Autodesk Inventor part; units mm, degrees
ref_plane "YZ Plane" through (0, 0, 0) normal (1, 0, 0) x (0, 1, 0)
ref_plane "XZ Plane" through (0, 0, 0) normal (0, 1, 0) x (-1, 0, 0)
ref_plane "XY Plane" through (0, 0, 0) normal (0, 0, 1) x (1, 0, 0)
sketch "Sketch1" plane through (0, 0, 0) normal (0, 0, 1) x (1, 0, 0)
  line L0 (-212.471, -44.069) -> (212.471, -44.069)
  line L1 (212.471, -44.069) -> (212.471, 44.069)
  line L2 (212.471, 44.069) -> (-212.471, 44.069)
  line L3 (-212.471, 44.069) -> (-212.471, -44.069)
  line L4 (-212.471, -44.069) -> (212.471, 44.069) construction
  line L5 (212.471, -44.069) -> (-212.471, 44.069) construction
  point P0 (0, 0)
  dimension "d0" = 424.942
  dimension "d1" = 88.138
extrude "Extrusion1" add sketch "Sketch1" along normal blind 1.651
sketch "SMA" plane through (0, 0, 1.651) normal (0, 0, 1) x (1, 0, 0)
  line L0 (-209.423, -35.814) -> (209.423, -35.814) construction
  line L1 (209.423, -35.814) -> (209.423, 35.814) construction
  line L2 (209.423, 35.814) -> (-209.423, 35.814) construction
  line L3 (-209.423, 35.814) -> (-209.423, -35.814) construction
  line L4 (212.471, 44.069) -> (-212.471, 44.069) construction
  line L5 (212.471, -44.069) -> (212.471, 44.069) construction
  line L6 (-212.471, 44.069) -> (-212.471, -44.069)
  line L7 (-212.471, -44.069) -> (212.471, -44.069)
  line L8 (-222.5982, 0) -> (228.0899, 0) construction
  line L9 (0, 79.8165) -> (0, -88.5526) construction
  line L10 (-181.2798, 19.5533) -> (-181.2798, 0.2592) construction
  line L11 (-189.2532, 10.414) -> (-170.7489, 10.414) construction
  arc A0 (-184.023, 8.669) -> (-184.023, 12.159) centre (-181.2798, 10.414) ccw
  line L12 (-184.023, 12.159) -> (-184.023, 8.669)
  line L13 (-145.923, 12.159) -> (-145.923, 8.669)
  arc A1 (-145.923, 8.669) -> (-145.923, 12.159) centre (-143.1798, 10.414) ccw
  line L14 (-184.023, -13.241) -> (-184.023, -16.731)
  arc A2 (-184.023, -16.731) -> (-184.023, -13.241) centre (-181.2798, -14.986) ccw
  line L15 (-145.923, -13.241) -> (-145.923, -16.731)
  arc A3 (-145.923, -16.731) -> (-145.923, -13.241) centre (-143.1798, -14.986) ccw
  line L16 (-120.523, 12.159) -> (-120.523, 8.669)
  arc A4 (-120.523, 8.669) -> (-120.523, 12.159) centre (-117.7798, 10.414) ccw
  arc A5 (-120.523, -16.731) -> (-120.523, -13.241) centre (-117.7798, -14.986) ccw
  line L17 (-120.523, -13.241) -> (-120.523, -16.731)
  line L18 (-95.123, 12.159) -> (-95.123, 8.669)
  arc A6 (-95.123, 8.669) -> (-95.123, 12.159) centre (-92.3798, 10.414) ccw
  arc A7 (-95.123, -16.731) -> (-95.123, -13.241) centre (-92.3798, -14.986) ccw
  line L19 (-95.123, -13.241) -> (-95.123, -16.731)
  line L20 (-69.723, 12.159) -> (-69.723, 8.669)
  arc A8 (-69.723, 8.669) -> (-69.723, 12.159) centre (-66.9798, 10.414) ccw
  arc A9 (-69.723, -16.731) -> (-69.723, -13.241) centre (-66.9798, -14.986) ccw
  line L21 (-69.723, -13.241) -> (-69.723, -16.731)
  point P0 (0, 0)
  point P1 (-178.0286, 10.414)
  point P2 (-139.9286, 10.414)
  point P3 (-178.0286, -14.986)
  point P4 (-139.9286, -14.986)
  point P5 (-114.5286, 10.414)
  point P6 (-114.5286, -14.986)
  point P7 (-89.1286, 10.414)
  point P8 (-89.1286, -14.986)
  point P9 (-63.7286, 10.414)
  point P10 (-63.7286, -14.986)
  point P11 (-63.7286, -14.986)
  dimension "d4" = 8.255
  dimension "d5" = 3.048
  dimension "d7" = 8.255
  dimension "d8" = 3.048
  dimension "d11" = 6.5024
  dimension "d12" = 5.9944
  dimension "d13" = 25.4
  dimension "d14" = 25.4
  dimension "d17" = 38.1
  dimension "d20" = 25.4
  dimension "d25" = 25.4
sketch "airflow" plane through (0, 0, 1.651) normal (0, 0, 1) x (1, 0, 0)
  line L0 (146.685, -25.019) -> (196.723, -25.019) construction
  line L1 (196.723, -25.019) -> (196.723, 25.019) construction
  line L2 (196.723, 25.019) -> (146.685, 25.019) construction
  line L3 (146.685, 25.019) -> (146.685, -25.019) construction
  line L4 (146.685, -25.019) -> (196.723, 25.019) construction
  line L5 (196.723, -25.019) -> (146.685, 25.019) construction
  line L6 (209.423, -35.814) -> (209.423, 35.814) construction
  line L7 (209.423, 35.814) -> (-209.423, 35.814) construction
  line L8 (-209.423, -35.814) -> (209.423, -35.814) construction
  line L9 (-209.423, 35.814) -> (-209.423, -35.814) construction
  line L10 (-212.471, -44.069) -> (212.471, -44.069)
  line L11 (212.471, -44.069) -> (212.471, 44.069)
  line L12 (212.471, 44.069) -> (-212.471, 44.069)
  line L13 (-212.471, 44.069) -> (-212.471, -44.069)
  line L14 (150.6195, -21.0845) -> (192.7885, -21.0845)
  line L15 (192.7885, -21.0845) -> (192.7885, 21.0845)
  line L16 (192.7885, 21.0845) -> (150.6195, 21.0845)
  line L17 (150.6195, 21.0845) -> (150.6195, -21.0845)
  line L18 (150.6195, -21.0845) -> (192.7885, 21.0845) construction
  line L19 (192.7885, -21.0845) -> (150.6195, 21.0845) construction
  point P0 (171.704, 0)
  point P1 (252.5868, -10.4776)
  dimension "d30" = 50.038
  dimension "d31" = 50.038
  dimension "d32" = 12.7
  dimension "d218" = 3.9345
  dimension "d229" = 44.069
sketch "Dsub25" plane through (0, 0, 1.651) normal (0, 0, 1) x (1, 0, 0)
  line L0 (78.613, 20.0279) -> (78.613, -20.0279)
  line L1 (66.929, 18.4404) -> (66.929, -18.4404)
  arc A0 (76.1166, -22.0536) -> (78.613, -20.0279) centre (76.5429, -20.0279) ccw
  arc A1 (66.929, -18.4404) -> (68.5728, -20.4661) centre (68.9991, -18.4404) ccw
  arc A2 (78.613, 20.0279) -> (76.1166, 22.0536) centre (76.5429, 20.0279) ccw
  arc A3 (68.5728, 20.4661) -> (66.929, 18.4404) centre (68.9991, 18.4404) ccw
  line L2 (49.6457, 0) -> (87.8983, 0) construction
  line L3 (-212.471, -44.069) -> (212.471, -44.069) construction
  line L4 (72.771, 23.5839) -> (72.771, -23.5839) construction
  line L5 (76.1166, 22.0536) -> (68.5728, 20.4661)
  line L6 (76.1166, -22.0536) -> (68.5728, -20.4661)
  line L7 (-212.471, 44.069) -> (-212.471, -44.069)
  point P0 (0, 0)
  point P1 (78.613, 0)
  point P2 (66.929, 0)
  point P3 (72.771, 0)
  point P4 (72.771, 21.3496)
  dimension "d46" = 47.1678
  dimension "d47" = 4.1402
  dimension "d48" = 4.1402
  dimension "d49" = 4.1402
  dimension "d50" = 4.1402
  dimension "d51" = 40.0558
  dimension "d52" = 36.8808
  dimension "d53" = 44.069
  dimension "d57" = 11.684
  dimension "d58" = 5.842
  dimension "d59" = 279.4
  dimension "d60" = 44.069
extrude "sma cutouts" cut sketch "SMA" against normal through all
hole "dsub25 holes" at (72.771, 23.5839, 1.651) at (72.771, -23.5839, 1.651) direction (0, 0, -1) diameter 2.9464 end through all
extrude "dsub25 cutout" cut sketch "Dsub25" against normal through all
sketch "rj45" plane through (0, 0, 1.651) normal (0, 0, 1) x (1, 0, 0)
  line L0 (-47.371, 3.429) -> (-30.226, 3.429)
  line L1 (-30.226, 3.429) -> (-30.226, 26.289)
  line L2 (-30.226, 26.289) -> (-47.371, 26.289)
  line L3 (-47.371, 26.289) -> (-47.371, 3.429)
  line L4 (-47.371, 3.429) -> (-30.226, 26.289) construction
  line L5 (-30.226, 3.429) -> (-47.371, 26.289) construction
  line L6 (-38.7985, 29.337) -> (-38.7985, 0.381) construction
  line L7 (-212.471, 44.069) -> (-212.471, -44.069) construction
  line L8 (212.471, 44.069) -> (-212.471, 44.069) construction
  line L9 (3.429, 3.429) -> (20.574, 3.429)
  line L10 (20.574, 3.429) -> (20.574, 26.289)
  line L11 (20.574, 26.289) -> (3.429, 26.289)
  line L12 (3.429, 26.289) -> (3.429, 3.429)
  line L13 (3.429, 3.429) -> (20.574, 26.289) construction
  line L14 (20.574, 3.429) -> (3.429, 26.289) construction
  line L15 (12.0015, 29.337) -> (12.0015, 0.381) construction
  line L16 (-21.971, -25.527) -> (-4.826, -25.527)
  line L17 (-4.826, -25.527) -> (-4.826, -2.667)
  line L18 (-4.826, -2.667) -> (-21.971, -2.667)
  line L19 (-21.971, -2.667) -> (-21.971, -25.527)
  line L20 (-21.971, -25.527) -> (-4.826, -2.667) construction
  line L21 (-4.826, -25.527) -> (-21.971, -2.667) construction
  line L22 (-13.3985, 0.381) -> (-13.3985, -28.575) construction
  line L23 (28.829, -25.527) -> (45.974, -25.527)
  line L24 (45.974, -25.527) -> (45.974, -2.667)
  line L25 (45.974, -2.667) -> (28.829, -2.667)
  line L26 (28.829, -2.667) -> (28.829, -25.527)
  line L27 (28.829, -25.527) -> (45.974, -2.667) construction
  line L28 (45.974, -25.527) -> (28.829, -2.667) construction
  line L29 (37.4015, 0.381) -> (37.4015, -28.575) construction
  line L30 (-212.471, -44.069) -> (212.471, -44.069) construction
  line L31 (-38.7985, 0.381) -> (62.2062, 0.381) construction
  point P0 (0, 0)
  point P1 (-38.7985, 14.859)
  point P2 (-38.7985, 14.859)
  point P3 (12.0015, 14.859)
  point P4 (12.0015, 14.859)
  point P5 (-13.3985, -14.097)
  point P6 (-13.3985, -14.097)
  point P7 (37.4015, -14.097)
  point P8 (37.4015, -14.097)
  dimension "d160" = 28.956
  dimension "d161" = 22.86
  dimension "d162" = 17.145
  dimension "d163" = 165.1
  dimension "d164" = 17.78
  dimension "d165" = 28.956
  dimension "d166" = 22.86
  dimension "d167" = 17.145
  dimension "d168" = 28.956
  dimension "d169" = 22.86
  dimension "d170" = 17.145
  dimension "d171" = 28.956
  dimension "d172" = 22.86
  dimension "d173" = 17.145
  dimension "d174" = 17.78
  dimension "d175" = 215.9
  dimension "d177" = 190.5
  dimension "d179" = 241.3
hole "rj45 holes" at (-38.7985, 29.337, 1.651) at (-38.7985, 0.381, 1.651) at (12.0015, 0.381, 1.651) at (12.0015, 29.337, 1.651) at (-13.3985, -28.575, 1.651) at (-13.3985, 0.381, 1.651) at (37.4015, -28.575, 1.651) at (37.4015, 0.381, 1.651) direction (0, 0, -1) diameter 3.2766 end through all
extrude "rj45 cutouts" cut sketch "rj45" against normal blind 25.4
sketch "rj45 debug" plane through (0, 0, 1.651) normal (0, 0, 1) x (1, 0, 0)
  line L0 (101.5365, 3.429) -> (118.6815, 3.429)
  line L1 (118.6815, 3.429) -> (118.6815, 26.289)
  line L2 (118.6815, 26.289) -> (101.5365, 26.289)
  line L3 (101.5365, 26.289) -> (101.5365, 3.429)
  line L4 (101.5365, 3.429) -> (118.6815, 26.289) construction
  line L5 (118.6815, 3.429) -> (101.5365, 26.289) construction
  line L6 (110.109, 29.337) -> (110.109, 0.381) construction
  line L7 (-212.471, 44.069) -> (-212.471, -44.069)
  line L8 (212.471, 44.069) -> (-212.471, 44.069)
  point P0 (0, 0)
  point P1 (110.109, 14.859)
  point P2 (110.109, 14.859)
  dimension "d189" = 28.956
  dimension "d190" = 17.145
  dimension "d191" = 22.86
  dimension "d193" = 17.78
  dimension "d194" = 322.58
hole "rj45 debug holes" at (110.109, 29.337, 1.651) at (110.109, 0.381, 1.651) direction (0, 0, -1) diameter 3.2766 end through all
extrude "rj45 debug cutout" cut sketch "rj45 debug" against normal blind 25.4
sketch "SC/SC" plane through (0, 0, 1.651) normal (0, 0, 1) x (1, 0, 0)
  line L0 (103.632, -16.1798) -> (116.586, -16.1798)
  line L1 (116.586, -16.1798) -> (116.586, -25.527)
  line L2 (116.586, -25.527) -> (103.632, -25.527)
  line L3 (103.632, -25.527) -> (103.632, -16.1798)
  line L4 (103.632, -16.1798) -> (116.586, -25.527) construction
  line L5 (116.586, -16.1798) -> (103.632, -25.527) construction
  line L6 (101.109, -20.8534) -> (119.109, -20.8534) construction
  line L7 (-212.471, 44.069) -> (-212.471, -44.069)
  line L8 (-212.471, -44.069) -> (212.471, -44.069)
  point P0 (0, 0)
  point P1 (110.109, -20.8534)
  point P2 (110.109, -20.8534)
  dimension "d204" = 12.954
  dimension "d205" = 9.3472
  dimension "d206" = 18
  dimension "d207" = 322.58
  dimension "d208" = 18.542
hole "SC/SC holes" at (101.109, -20.8534, 1.651) at (119.109, -20.8534, 1.651) direction (0, 0, -1) diameter 2.3876 end through all
extrude "SC/SC cutout" cut sketch "SC/SC" against normal blind 25.4
hole "airflow holes" at (146.685, 25.019, 1.651) at (196.723, 25.019, 1.651) at (196.723, -25.019, 1.651) at (146.685, -25.019, 1.651) direction (0, 0, -1) diameter 5.1054 end through all
extrude "airflow cutout" cut sketch "airflow" against normal through all contours L17 L16 L15 L14
properties part number "nmt_frontpanel"
Can you work these out from the model? Positions are in its coordinate system, mm. Coordinates: 2 decimals unless noted, no trailing zeros. Loops run counter-clockwise (first coordinate to the right, second up) from the corner with the lowest first, then second, coordinate; pieces in that order, holes last. Notation, with made-up numbers: M 60.25,45 L 64.25,45 A16 ccw 64.25,75 Z; hole C 88.25,12.25 d2. An arc over 180 degrees is marked long. Return JSON: item names as keys, results as strings. Group by question number.
Item 1: Imagine slicing it at A-A (x = 156.5). Please give me the cut outline in (y, z).
Item 2: I'm going to push a flat-ended pin straight in: pin 1 Ø8.5 at (x, y) = (-117.78, 10.41) entering from -Z. Where does the tip first touch, or does it pass through?
Item 3: If I drill on L1, parallel to X at y = -10.5, z = 0.75; L2, parallel to X at y = -1.5, z = 0.95; L3, parallel to X at y = -19, z = 0.2, over which ranges is the centre line in solid material (lowest first)? Write a range as from..to.
Item 4: Imagine slicing it at B-B (z = 0.95). Give the number of separate pieces and of enclosed holes in the cut face, and give its area (3 significant figures).
Verdict:
{
 "1": {"outline": "M -44.07,0 L -21.08,0 L -21.08,1.65 L -44.07,1.65 Z; M 21.08,0 L 44.07,0 L 44.07,1.65 L 21.08,1.65 Z"},
 "2": {"pin 1": "stops at z = 0"},
 "3": {"L1": "x = -212.47..-21.97, -4.83..28.83, 45.97..66.93, 78.61..150.62, 192.79..212.47", "L2": "x = -212.47..66.93, 78.61..150.62, 192.79..212.47", "L3": "x = -212.47..-21.97, -4.83..28.83, 45.97..67.01, 78.61..103.63, 116.59..150.62, 192.79..212.47"},
 "4": {"separate pieces": "1", "enclosed holes": "36", "area": "32,600 mm^2"}
}
